Study the drawing (mm; zero at the part's minimum x, y, z) and answer. A direction names the side the tool comes from. Give positions to 0.01 mm unless a question says otherwise; leave off trailing zeros. Write each loop counter-clockwise with the first axis right and the second up, starting at its lowest first coordinate (ties: lowest second). Pieces come first, ordered by that corner, then holes. Notation, with made-up numbers: (-17, 17) - (10, 17) arc R14 ccw to (10, 34) - close; hole circle Ø6 at (5.25, 21.5). An arc over 180 degrees is marked (long way). Write each question's results on one line, items separated by ' | '. Start each with the question number.
Q1. Section D-D (y = 23) is taken. Determine the outline of the cut face in (x, z).
Q2. Flat-ended cylindrical pins translate along their axes: pin 1 Ø1.5 at (x, z) = (54, 47) entering from +Y; pin 2 Ø10 at (y, z) = (39.5, 27.5) entering from -X (1 decimal); pin 3 Ø12 at (x, z) = (26.5, 15.5) entering from +Y (1 decimal). Find the tip coordinate at first contact, or state that the pin passes through.
Q3. For a pull along Z with two mould halves and no side action, classify the marked faces 1, 2 and 3 as pulls with the +Z half, pulls with the -Z half, needs draft (parallel to the pull), parting line crosses it, or undercut.
Q4. Section A-A (z = 38) is taken. Determine the outline of the cut face in (x, y) (1 decimal), plus the area to 3 significant figures.
Q5. Section B-B (x = 38) is taken. Determine the outline of the cut face in (y, z) (1 decimal), plus the area to 3 significant figures.
Q6. For the marked faces 4 and 5, determine the directions among +Z, -Z, +X, -X, +Y, -Y from which every point of the face is accessible in a straight line to the end or side of a thin tool.
Q7. Find the intervals of material crossed by probe 1 along Z at (x, y) = (38, 1.6); probe 2 along X at (y, z) = (4.5, 37) (1 decimal); probe 3 along Y at (x, z) = (38.5, 42), in increasing order.
Q8. Section C-C (y = 67) is taken. Determine the outline of the cut face in (x, z).
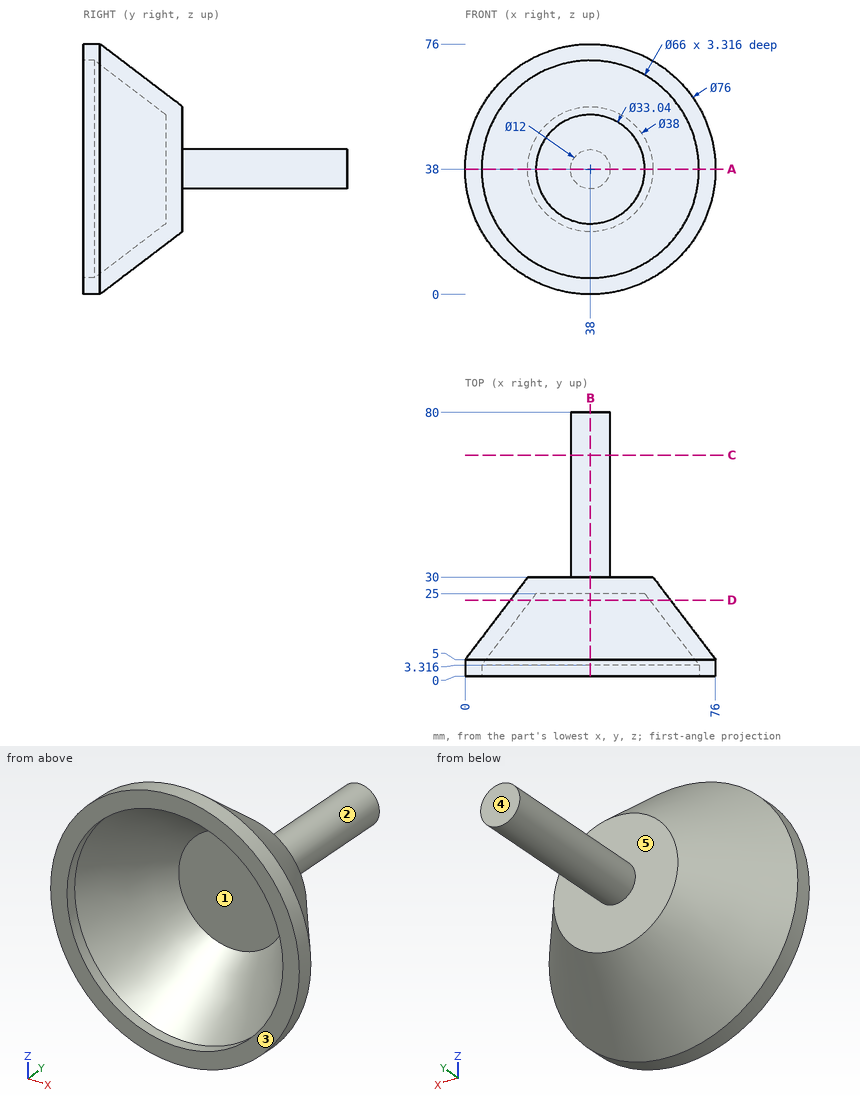
Answers below:
1) outline: circle Ø48.64 at (38, 38); hole circle Ø36.08 at (38, 38)
2) pin 1: stops at y = 30 | pin 2: stops at x = 35.6 | pin 3: stops at y = 29.6
3) face 1: undercut | face 2: parting line crosses it | face 3: needs draft
4) outline: (0, 0) - (5, 0) - (5, 3.3) - (21.5, 25) - (54.5, 25) - (71, 3.3) - (71, 0) - (76, 0) - (76, 5) - (57, 30) - (44, 30) - (44, 80) - (32, 80) - (32, 30) - (19, 30) - (0, 5) - close | area: 1,110 mm2
5) outline: (0, 0) - (5, 0) - (30, 19) - (30, 32) - (80, 32) - (80, 44) - (30, 44) - (30, 57) - (5, 76) - (0, 76) - (0, 71) - (3.3, 71) - (25, 54.5) - (25, 21.5) - (3.3, 5) - (0, 5) - close | area: 1,110 mm2
6) face 4: +Z, -Z, +X, -X, +Y | face 5: +Y
7) probe 1: z = 0 to 5, 71 to 76 | probe 2: x = 0 to 5.9, 70.1 to 76 | probe 3: y = 25 to 80
8) outline: circle Ø12 at (38, 38)
